Check sheet for the drawn part. Datum: minimum x, y, z corner. Units: mm. Give positions to 0.01 mm unless a question says otherwise; leave off trailing zeros. Order: outer loops, then holes, each group sorted by start corner. A loop starts at its lowest first (then second) coordinate and runs counter-clockwise, first axis right, second up. Notation, with made-up numbers: (-27, 16) - (15, 16) arc R18 ccw to (15, 28) - close; hole circle Ø7 at (-5.5, 13). An arc over 180 degrees is marked (long way). Answer as a JSON object with one key per item and string values. Group by question number.
(1) Depth check by flat-ended pin: pin 1 Ø17 at (x, z) = (15.875, 15.875) entering from +Y; pin 2 Ø4 at (y, z) = (97.5, 25) entering from -X; pin 3 Ø5 at (x, y) = (20.5, 73.5) entering from +Z; pin 4 Ø12 at (x, y) = (3.5, 109) entering from +Z. Enter the tip coordinate at first touch or a pass-through.
(2) Section check B-B (z = 24). Record the boundary of the cut face in (x, y), then the cut area to 3 significant figures.
(3) Section check A-A (x = 12). Record the boundary of the cut face in (y, z).
(4) Thickness scan on line 1 (Z direction, x = 9.5, y = 99.5); line 2 (Z direction, x = 14, y = 88.5); line 3 (X direction, y = 111.5, z = 17.5). Record the ranges inside material, lowest first.
(5) Mould release check, pull along X, two halves, no side actions. Record for the marked faces 1 and 2: +X half, -X half, draft (parallel to the pull), parting line (faces both ways), or undercut.
(6) Section check D-D (x = 3.5). Record the boundary of the cut face in (y, z), then the cut area to 3 significant figures.
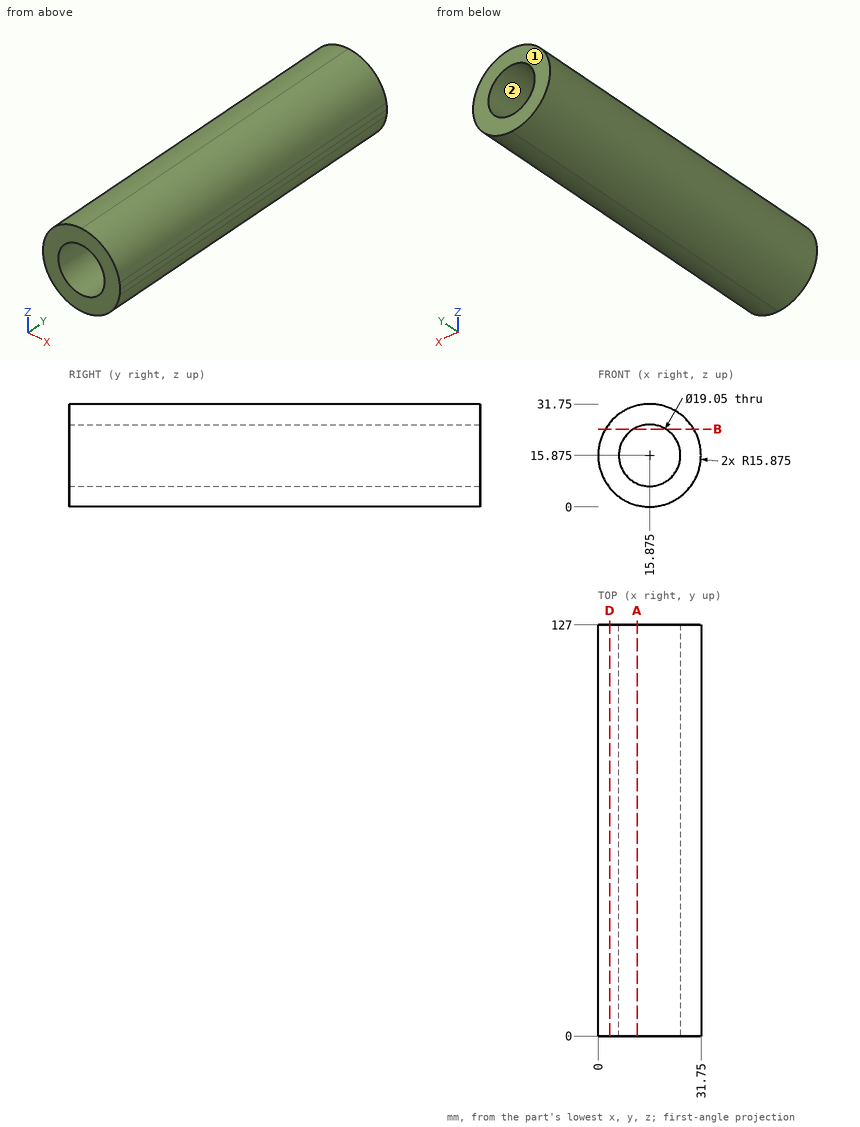
Solutions:
{
 "1": {"pin 1": "passes through", "pin 2": "stops at x = 1.69", "pin 3": "stops at z = 31.61", "pin 4": "stops at z = 30.41"},
 "2": {"outline": "(2.24, 0) - (10.9, 0) - (10.9, 127) - (2.24, 127) - close; (20.85, 0) - (29.51, 0) - (29.51, 127) - (20.85, 127) - close", "area": "2,200 mm2"},
 "3": {"outline": "(0, 0.48) - (127, 0.48) - (127, 7.17) - (0, 7.17) - close; (0, 24.58) - (127, 24.58) - (127, 31.27) - (0, 31.27) - close"},
 "4": {"line 1": "z = 1.34 to 8.8, 22.95 to 30.41", "line 2": "z = 0.11 to 6.54, 25.21 to 31.64", "line 3": "x = 0.08 to 6.49, 25.26 to 31.67"},
 "5": {"face 1": "draft", "face 2": "undercut"},
 "6": {"outline": "(0, 5.93) - (127, 5.93) - (127, 25.82) - (0, 25.82) - close", "area": "2,530 mm2"}
}
